from build123d import *

# Parameters (mm, degrees)
ESQUISSE1_R                  = 5
BOSS_EXTRU_1_DEPTH           = 50
ENL_V_MAT_EXTRU_1_DEPTH      = 16
ENL_V_MAT_EXTRU_1_DEPTH_BACK = 16
ENL_V_MAT_EXTRU_2_REACH      = 52


with BuildPart() as part:
    # Esquisse1 → Boss.-Extru.1 (new body)
    with BuildSketch(Plane.XY):
        with BuildLine():
            Line((-15, -17.5), (15, -17.5))
            Line((15, -17.5), (15, 17.5))
            ThreePointArc((15, 17.5), (0, 32.5), (-15, 17.5))
            Line((-15, 17.5), (-15, -17.5))
        make_face()
        with Locations((0, 17.5)):
            Circle(ESQUISSE1_R, mode=Mode.SUBTRACT)
    extrude(amount=-BOSS_EXTRU_1_DEPTH)

    # Esquisse2 → Enlèv. mat.-Extru.1 (cut, two sides)
    with BuildSketch(Plane(origin=(0, 0, 0), x_dir=(0, 0, -1), z_dir=(1, 0, 0))) as enl_v_mat_extru_1_sk:
        Polygon((0, -17.5), (10, 32.5), (0, 32.5), align=None)
    extrude(amount=ENL_V_MAT_EXTRU_1_DEPTH, mode=Mode.SUBTRACT)
    extrude(enl_v_mat_extru_1_sk.sketch, amount=-ENL_V_MAT_EXTRU_1_DEPTH_BACK, mode=Mode.SUBTRACT)

    # Enlèv. mat.-Extru.2: up to this plane
    enl_v_mat_extru_2_end = Plane(origin=(-15, -17.89223227, -1.961161351), z_dir=(0, -0.196116135, -0.980580676))
    # Esquisse3 → Enlèv. mat.-Extru.2 (cut, up to the surface)
    with BuildSketch(Plane(origin=(0, 0, -50), x_dir=(-1, 0, 0), z_dir=(0, 0, -1)), mode=Mode.PRIVATE) as enl_v_mat_extru_2_sk1:
        with BuildLine():
            Line((-13, 17.5), (-13, -15.5))
            Line((-13, -15.5), (13, -15.5))
            Line((13, -15.5), (13, 17.5))
            ThreePointArc((13, 17.5), (0, 30.5), (-13, 17.5))
        make_face()
    enl_v_mat_extru_2_tool1 = split(extrude(enl_v_mat_extru_2_sk1.sketch, amount=-ENL_V_MAT_EXTRU_2_REACH, mode=Mode.PRIVATE), bisect_by=enl_v_mat_extru_2_end, keep=Keep.BOTH, mode=Mode.PRIVATE)
    add(enl_v_mat_extru_2_tool1.solids().sort_by_distance((0, 6.202507, -50))[0], mode=Mode.SUBTRACT)


solid = part.part
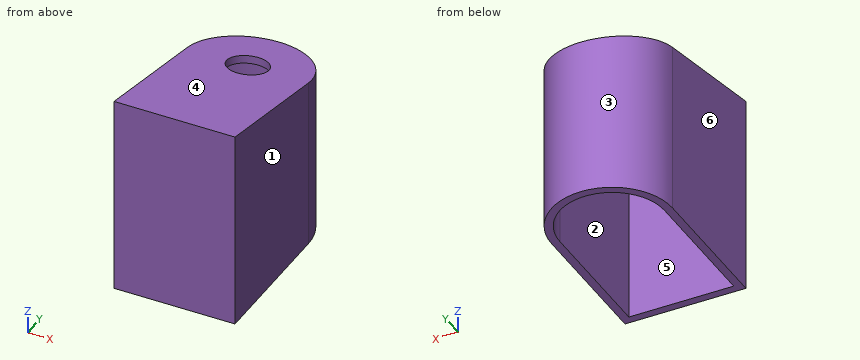
Here's how the part is built. I have some questions about the finished solid (model axes, mm). Face numbers are marked on the shaded views. A direction names the side the tool comes from. Give positions to 0.01 mm unless a question says otherwise; leave off trailing zeros. Order: outer loops, then holes, each group sorted by start corner. A loop starts at its lowest first (then second) coordinate and runs counter-clockwise, first axis right, second up. Notation, with made-up numbers: (60, 39.5) -> (88, 39.5) arc R19 cw to (88, 76.5) -> close; hole circle Ø4 at (82.25, 25). An arc over 180 degrees is marked (long way). Use a Markdown table: item, result. Add a question column.
Item 1: Imagine slicing it at C-C on y = 1. Please give me the cut outline in (x, z), plus the area to 3 significant figures.
Item 2: If we mould it in two halves opening along X, with no side actions, what happens to the marked faces 3, 4, 5 and 6? For each: pulls with the +X half, pulls with the -X half, needs draft (parallel to the pull), parting line crosses it, or undercut.
Item 3: Imagine slicing it at A-A on z = -41. Please give me the cut outline in (x, y).
Item 4: Imagine slicing it at D-D on x = 8.5. Please give me the cut outline in (y, z).
Item 5: I need wall thicknesses on line 1 (X direction, y = 17, z = -13); line 2 (X direction, y = 17.5, z = -8.9); line 3 (Y direction, x = 12, z = -20.5). Which ranges of each line are inside material? Lowest first, please.
Item 6: Imagine slicing it at B-B on x = 0. Please give me the cut outline in (y, z).
Item 7: For the marked faces 1 and 2, which set-ups out of +Z, -Z, +X, -X, +Y, -Y let a thin tool reach every point of the face, with its end or its side?
Item 8: Will these pins go through, and if not, where does the flat tip stop? pin 1 (11.5 mm diameter, centred on x = 0, y = 17.5, fed in from +Z); pin 2 (2 mm diameter, centred on x = -5, z = -26.5, fed in from +Y); pin 3 (4 mm diameter, centred on y = 24.5, z = -32.5, fed in from +X).
Data:
| question | item | result |
|---|---|---|
| 1 | outline | (-15, -50) -> (-13, -50) -> (-13, -5.74) -> (13, -5.74) -> (13, -50) -> (15, -50) -> (15, -3.7) -> (-15, -3.7) -> close |
| 1 | area | 238 mm² |
| 2 | face 3 | parting line crosses it |
| 2 | face 4 | needs draft |
| 2 | face 5 | undercut |
| 2 | face 6 | pulls with the -X half |
| 3 | outline | (-15, -17.5) -> (15, -17.5) -> (15, 17.5) arc R15 ccw to (-15, 17.5) -> close; hole (-13, -15.5) -> (13, -15.5) -> (13, 17.5) arc R13 ccw to (-13, 17.5) -> close |
| 4 | outline | (-17.5, -50) -> (-15.5, -50) -> (-15.5, -2.44) -> (27.34, -11.01) -> (27.34, -50) -> (29.86, -50) -> (29.86, -9.47) -> (-17.5, 0) -> close |
| 5 | line 1 | x = -15 to -13, 13 to 15 |
| 5 | line 2 | x = -15 to -5, 5 to 15 |
| 5 | line 3 | y = -17.5 to -15.5, 22.5 to 26.5 |
| 6 | outline | (-17.5, -50) -> (-15.5, -50) -> (-15.5, -2.44) -> (12.5, -8.04) -> (12.5, -6) -> (-17.5, 0) -> close; (22.5, -10.04) -> (30.5, -11.64) -> (30.5, -50) -> (32.5, -50) -> (32.5, -10) -> (22.5, -8) -> close |
| 7 | face 1 | +Z, -Z, +X, +Y, -Y |
| 7 | face 2 | -Z |
| 8 | pin 1 | stops at z = -5.85 |
| 8 | pin 2 | stops at y = 31.96 |
| 8 | pin 3 | stops at x = 14.14 |
